Source: CAD feature listing. Evaluate the final solid. Frame: model axes, mm. A direction names the side the tool comes from. Give positions to 0.01 mm unless a question says otherwise; leave off trailing zeros. Loops run counter-clockwise (first coordinate to the right, second up) from the corner with the lowest first, then second, coordinate; pieces in that order, holes last. Notation, with made-up numbers: (70.25, 58) - (120.25, 58) arc R22 ccw to (120.25, 72) - close; hole circle Ø9 at (-15.75, 82.5). An arc over 180 degrees is marked (long way). Put each result on its own line as item: value.
```python
from build123d import *

# Parameters (mm, degrees)
F1_DEPTH = 8
F2_R     = 3
F4_DEPTH = 5


with BuildPart() as f1:
    # F0 (on Top) → F1 (new body)
    with BuildSketch(Plane.XY):
        with BuildLine():
            ThreePointArc((5, 0), (1.4644660941, -1.4644660941), (0, -5))
            Line((0, -5), (0, -35))
            ThreePointArc((0, -35), (2.9289321881, -42.0710678119), (10, -45))
            Line((10, -45), (40, -45))
            ThreePointArc((40, -45), (43.5355339059, -43.5355339059), (45, -40))
            Line((45, -40), (45, -35))
            ThreePointArc((45, -35), (43.5355339059, -31.4644660941), (40, -30))
            Line((40, -30), (15, -30))
            Line((15, -30), (15, -5))
            ThreePointArc((15, -5), (13.5355339059, -1.4644660941), (10, 0))
            Line((10, 0), (5, 0))
        make_face()
    extrude(amount=F1_DEPTH)

    # F2
    f2_edges = [f1.edges().sort_by_distance(p)[0] for p in [
        (15, -17.5, 8),
        (27.5, -30, 8),
        (13.535534, -1.464466, 8),
        (7.5, 0, 8),
        (1.464466, -1.464466, 8),
        (0, -20, 8),
        (2.928932, -42.071068, 8),
        (25, -45, 8),
        (43.535534, -43.535534, 8),
        (45, -37.5, 8),
        (43.535534, -31.464466, 8),
    ]]
    fillet(f2_edges, radius=F2_R)

    # F3 (on face) → F4 (join)
    with BuildSketch(Plane(origin=(0, 0, 0), x_dir=(1, 0, 0), z_dir=(0, 0, -1))):
        with BuildLine():
            ThreePointArc((7.5502525317, 37.4497474683), (7.5502525317, 34.6213203436), (10.3786796564, 34.6213203436))
            Line((10.3786796564, 34.6213203436), (7.5502525317, 37.4497474683))
        make_face()
        with BuildLine():
            Line((7.5502525317, 37.4497474683), (10.3786796564, 34.6213203436))
            ThreePointArc((10.3786796564, 34.6213203436), (10.8122251591, 35.2701670412), (10.9644660941, 36.0355339059))
            ThreePointArc((10.9644660941, 36.0355339059), (9.7298329588, 37.883292971), (7.5502525317, 37.4497474683))
        make_face()
    extrude(amount=F4_DEPTH)


solid = f1.part
```
1) Pin query (flat end, axial travel): P1, Ø5.5, axis at y = -23.5, z = 2.5, coming from the +X side; P2, Ø6, axis at y = -19, z = 6, coming from the -X side; P3, Ø2.5, axis at x = 21.5, z = 3.5, coming from the +Y side; P4, Ø13.5, axis at x = 17.5, y = -23, coming from the -Z side. Return the tip coordinate at first contact, or that it passes through.
Check result:
P1: x = 15
P2: x = 0
P3: y = -30
P4: z = 0
2) Section query C-C, the plane y = -17.5. Output: boundary loops of the cut face in (x, z).
Check result:
outline: (0, 0) - (15, 0) - (15, 5) arc R3 ccw to (12, 8) - (3, 8) arc R3 ccw to (0, 5) - close
3) Section query B-B, the plane z = 3.5. Output: boundary loops of the cut face in (x, y).
Check result:
outline: (0, -35) arc R10 ccw to (10, -45) - (40, -45) arc R5 ccw to (45, -40) - (45, -35) arc R5 ccw to (40, -30) - (15, -30) - (15, -5) arc R5 ccw to (10, 0) - (5, 0) arc R5 ccw to (0, -5) - close
4) Section query A-A, the plane x = 28.5. Output: boundary loops of the cut face in (y, z), plus the area to 3 significant figures.
Check result:
outline: (-45, 0) - (-30, 0) - (-30, 5) arc R3 ccw to (-33, 8) - (-42, 8) arc R3 ccw to (-45, 5) - close
area: 116 mm²
5) Material intervals for line 1 along Y through (x, z) = (16.5, 3.25); line 2 along Z through (x, y) = (4.5, -23.5); line 3 along X through (y, z) = (-21, 0.5), sorted ascending. Write a range as [from, to].
Check result:
line 1: [-45, -30]
line 2: [0, 8]
line 3: [0, 15]
6) Section query D-D, the plane z = -2.25. Output: boundary loops of the cut face in (x, y).
Check result:
outline: circle Ø4 at (8.96, -36.04)
7) Access query for faces 1 (the cylindrical face through (14.14, -18.8, 7.1)), 2 (the flat face through (15, -18, 2)), 3 (the cylindrical face through (0.86, -20.21, 7.1)). Directions: +Z, -Z, +X, -X, +Y, -Y. A direction counts if a zero-diameter tool reaches every point of the face in a straight line with its end or side. Return the directions, or none.
Check result:
face 1: +Z, +X, +Y
face 2: +Z, -Z, +X, +Y
face 3: +Z, -X, +Y, -Y
